Check sheet for the drawn part. Datum: minimum x, y, z corner. Units: mm. A direction names the side the tool comes from. Coordinates: 2 decimals unless noted, no trailing zeros. Write each loop counter-clockwise with the first axis right and the second up, starting at its lowest first coordinate (ties: lowest second). Pieces come first, ordered by that corner, then holes. Notation, with made-up numbers: M -17,50.5 L 3,50.5 A5 ccw 3,59.5 Z; hole C 12.5,73 d8. An arc over 180 degrees is marked long. Answer as CSV lines item,"result". Start each with the question number.
Q1. Sectioned sample at D-D, the plane x = 29.5. Record the cut outline in (y, z).
Q2. Access from +Z, -Z, +X, -X, +Y, -Y to the whole of each face (thin tool, end or side, straight path). Record for the marked faces 4, 5, 6 and 7.
Q3. Sectioned sample at A-A, the plane y = 30.06. Record the cut outline in (x, z) (3 decimals), then the cut area to 4 significant figures.
Q4. Sectioned sample at C-C, the plane z = 45. Count the separate pieces of the cut face and the enclosed holes in it, then the cut area to 3 significant figures.
Q5. Sectioned sample at B-B, the plane x = 38. Record the cut outline in (y, z) (3 decimals), then the cut area to 3 significant figures.
Q6. Thickness scan on line 1 along Y through (x, z) = (33.3, 45) (1 decimal); line 2 along Z through (x, y) = (38, 30); line 3 along Y through (x, z) = (37.75, 45) (3 decimals). Record the ranges inside material, lowest first. Write a range as from..to.
Q7. Depth check by flat-ended pin: pin 1 Ø10 at (y, z) = (25.5, 46.5) entering from -X; pin 2 Ø6 at (x, y) = (25.5, 31.5) entering from -Z; pin 3 Ø8 at (x, y) = (35.5, 8.5) entering from -Z (3 decimals); pin 4 Ø10 at (y, z) = (85.5, 65.5) entering from -X. Enter the tip coordinate at first touch or a pass-through.
Q8. Mould release check, pull along Z, two halves, no side actions. Record for the marked faces 1, 2 and 3: pulls with the +Z half, pulls with the -Z half, needs draft (parallel to the pull), parting line crosses it, or undercut.
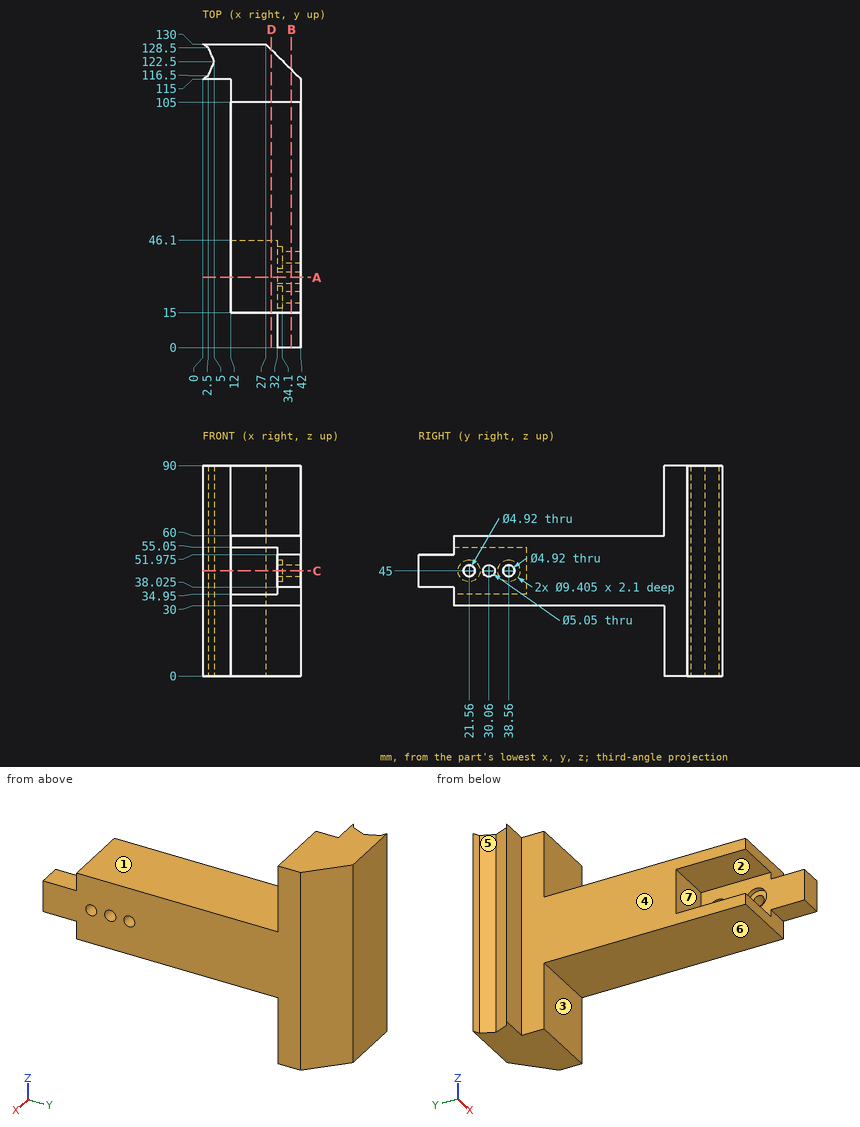
Output:
1,outline,"M 15,30 L 105,30 L 105,0 L 127.5,0 L 127.5,90 L 105,90 L 105,60 L 15,60 L 15,55.05 L 46.1,55.05 L 46.1,34.95 L 15,34.95 Z"
2,face 4,"+Z, -Z, -X, -Y"
2,face 5,"+Z, -Z, -X"
2,face 6,"-Z, +X, -X, -Y"
2,face 7,"-X, -Y"
3,outline,"M 12,30 L 42,30 L 42,42.475 L 32,42.475 L 32,34.95 L 12,34.95 Z; M 12,55.05 L 32,55.05 L 32,47.525 L 42,47.525 L 42,60 L 12,60 Z"
3,area,"447.5 mm^2"
4,separate pieces,"4"
4,enclosed holes,"0"
4,area,"2,830 mm^2"
5,outline,"M 0,38.025 L 15,38.025 L 15,30 L 105,30 L 105,0 L 119,0 L 119,90 L 105,90 L 105,60 L 15,60 L 15,51.975 L 0,51.975 Z; hole C 21.56,45 d4.92; hole C 30.06,45 d5.05; hole C 38.56,45 d4.92"
5,area,"4,110 mm^2"
6,line 1,"y = 0..16.9, 26.3..27.5, 32.6..33.9, 43.3..123.7"
6,line 2,"z = 30..42.48, 47.52..60"
6,line 3,"y = 0..19.1, 24.02..27.535, 32.585..36.1, 41.02..119.25"
7,pin 1,"stops at x = 32"
7,pin 2,"stops at z = 30"
7,pin 3,"stops at z = 38.025"
7,pin 4,"passes through"
8,face 1,"pulls with the +Z half"
8,face 2,"undercut"
8,face 3,"needs draft"
